Autodesk Inventor part; units mm, degrees
ref_plane "YZ Plane" through (0, 0, 0) normal (1, 0, 0) x (0, 1, 0)
ref_plane "XZ Plane" through (0, 0, 0) normal (0, 1, 0) x (-1, 0, 0)
ref_plane "XY Plane" through (0, 0, 0) normal (0, 0, 1) x (1, 0, 0)
sketch "Эскиз1" plane through (0, 0, 0) normal (0, 1, 0) x (-1, 0, 0)
  line L0 (0, 0) -> (14.1, 0)
  line L1 (14.1, 0) -> (14.1, -6)
  line L2 (14.1, -6) -> (0, -6)
  line L3 (0, -6) -> (0, 0)
  dimension "d0" = 14.1
  dimension "d1" = 6
extrude "Выдавливание1" add sketch "Эскиз1" along normal blind 13.15
sketch "Эскиз2" plane through (0, 13.15, 0) normal (0, 1, 0) x (1, 0, 0)
  line L0 (-14.1, 0) -> (0, 0)
  line L1 (-7.05, 0) -> (-7.05, 2.075)
  dimension "d4" = 2.075
hole "Отверстие1" at (-7.05, 13.15, -2.075) direction (0, -1, 0) diameter 2 depth 5 tip angle 118
sketch "Эскиз3" plane through (0, 0, 0) normal (0, -1, 0) x (1, 0, 0)
  line L0 (0, 0) -> (0, -6)
  line L1 (0, -3) -> (-3.05, -3)
  line L2 (-14.1, -6) -> (-14.1, 0)
  line L3 (-14.1, -3) -> (-11.05, -3)
  line L4 (0, 0) -> (0, -6)
  line L5 (-14.1, -6) -> (-14.1, 0)
  line L6 (-14.1, 0) -> (0, 0)
  dimension "d12" = 3
  dimension "d24" = 8
hole "Отверстие2" at (-3.05, 0, -3) at (-11.05, 0, -3) direction (0, 1, 0) diameter 2.2 depth 5
sketch "Эскиз4" plane through (0, 0, 0) normal (0, -1, 0) x (1, 0, 0)
  circle A0 centre (-3.05, -3) radius 1.1
  circle A1 centre (-11.05, -3) radius 1.1
  line L0 (-3.05, -5.2805) -> (-5.025, -4.1403)
  line L1 (-5.025, -4.1403) -> (-5.025, -1.8597)
  line L2 (-5.025, -1.8597) -> (-3.05, -0.7195)
  line L3 (-3.05, -0.7195) -> (-1.075, -1.8597)
  line L4 (-1.075, -1.8597) -> (-1.075, -4.1403)
  line L5 (-1.075, -4.1403) -> (-3.05, -5.2805)
  line L6 (0, 0) -> (0, -6)
  line L7 (-11.05, -5.2805) -> (-13.025, -4.1403)
  line L8 (-13.025, -4.1403) -> (-13.025, -1.8597)
  line L9 (-13.025, -1.8597) -> (-11.05, -0.7195)
  line L10 (-11.05, -0.7195) -> (-9.075, -1.8597)
  line L11 (-9.075, -1.8597) -> (-9.075, -4.1403)
  line L12 (-9.075, -4.1403) -> (-11.05, -5.2805)
  line L13 (-1.075, -1.8597) -> (-5.025, -1.8597)
  line L14 (-5.025, -1.8597) -> (-5.025, 0)
  line L15 (-5.025, 0) -> (-1.075, 0)
  line L16 (-1.075, 0) -> (-1.075, -1.8597)
  line L17 (-14.1, 0) -> (0, 0)
  line L18 (-9.075, -1.8597) -> (-13.025, -1.8597)
  line L19 (-13.025, -1.8597) -> (-13.025, 0)
  line L20 (-13.025, 0) -> (-9.075, 0)
  line L21 (-9.075, 0) -> (-9.075, -1.8597)
  point P0 (-3.05, 0)
  point P1 (-9.075, 0)
  dimension "d21" = 3.95
extrude "Выдавливание2" cut sketch "Эскиз4" along normal blind 2 from surface at -5 contours A0 | A1 | L21 L10 L9 L19 L17 | L0 L1 L13 L4 L5 | L14 L15 L16 L3 L2 | L2 L3 L13 | L18 L9 L10 | L11 L12 L7 L8 L18
chamfer "Фаска1" distance 0.8 distance2 6.15 1 edges at (-14.1, 13.15, -3) measured on face at (-7.05, 13.15, -5.025)
chamfer "Фаска2" distance 0.8 distance2 6.15 1 edges at (0, 13.15, -3) measured on face at (-6.7833, 13.15, -5.025)
chamfer "Фаска3" distance 1.5 distance2 6.15 1 edges at (-7.05, 13.15, -6) measured on face at (-7.05, 13.15, -5.025)
equation "\"Радиус_гибки\" = Толщина"
equation "\"Ширина_просечки\" = Толщина"
equation "\"Глубина_просечки\" = 0.5 * Толщина"
equation "\"Размер_просечки\" = 4 * Толщина"
equation "\"Мин_остаток\" = 2 * Толщина"
equation "\"Радиус_перехода\" = Радиус_гибки"
equation "\"Радиус_Якоби\" = Толщина"
equation "\"Размер_зазора\" = Толщина"
properties part number "Съемная стойка сервы"
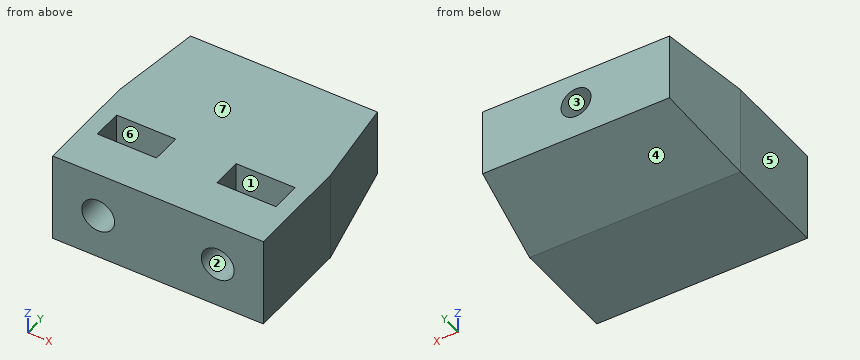
Read the model definition and answer for the solid it produces. Units are mm, in the model's axes. Face numbers are marked on the shaded views. A direction names the side the tool comes from. Coordinates: 2 decimals unless noted, no trailing zeros. Write each loop counter-clockwise with the first axis right and the second up, starting at its lowest first coordinate (ties: lowest second). Pieces come first, ordered by that corner, then holes. Notation, with made-up numbers: (-13.75, 4.25) - (0.25, 4.25) arc R20 cw to (0.25, 16.25) - close; hole circle Ø4 at (-30, -5.5). An arc over 180 degrees is marked (long way). One line per question, with ' | ' between items.
Q1. Find section C-C, the plane z = -4.75. Write down the section's boundary in (x, y) (3 decimals).
Result set:
outline: (-14.1, 0) - (0, 0) - (0, 7) - (-0.667, 12.125) - (-13.433, 12.125) - (-14.1, 7) - close; hole (-11.969, 3) - (-10.131, 3) - (-10.131, 5) - (-11.969, 5) - close; hole (-3.969, 3) - (-2.131, 3) - (-2.131, 5) - (-3.969, 5) - close
Q2. Consider L1, parallel to X at y = 1.9, z = -3; L2, parallel to Y at x = -4.75, z = -0.25; L3, parallel to Z at x = -11.05, y = 0.95. Determine where each line is inside the solid, lowest interval first. Write a range as [from, to].
Result set:
L1: [-14.1, -12.15], [-9.95, -4.15], [-1.95, 0] | L2: [0, 3], [5, 13.15] | L3: [-6, -4.1], [-1.9, 0]
Q3. Find section D-D, the plane y = 2.5. Write down the section's boundary in (x, z).
Result set:
outline: (-14.1, -6) - (0, -6) - (0, 0) - (-14.1, 0) - close; hole circle Ø2.2 at (-11.05, -3); hole circle Ø2.2 at (-3.05, -3)
Q4. For the marked faces 1, 2, 3 and 4, determine the directions among +Z, -Z, +X, -X, +Y, -Y from which every point of the face is accessible in a straight line to the end or side of a thin tool.
Result set:
face 1: +Z | face 2: -Y | face 3: +Y | face 4: -Z, +X, -X, +Y
Q5. Determine the mould class of the marked faces 5, 6 and 7 for opening direction X: +X half, -X half, draft (parallel to the pull), parting line (faces both ways), or undercut.
Result set:
face 5: -X half | face 6: undercut | face 7: draft
Q6. This flat-tipped pin is pushed along its axis until it touches: P1, Ø1.5, axis at y = 11, z = -2, coming from the -X side. Where does it stop, or does it pass through?
Result set:
P1: x = -13.68
Q7. Find section B-B, the plane x = -10.25. Write down the section's boundary in (y, z), plus the area to 3 significant figures.
Result set:
outline: (0, -6) - (7, -6) - (13.15, -4.5) - (13.15, 0) - (5, 0) - (5, -4.82) - (3, -4.82) - (3, -3.75) - (0, -3.75) - close; (0, -2.25) - (3, -2.25) - (3, 0) - (0, 0) - close | area: 60.1 mm^2
